Input: part model. Units: mm. Frame: model coordinates. A direction names the side the tool comes from. Give positions to 0.01 mm unless a question says otherwise; leave off trailing zeros. Write each loop counter-clockwise with the first axis right and the second up, starting at its lowest first coordinate (ties: lowest second). Pieces come first, ordered by that corner, then holes.
```python
from build123d import *

# Parameters (mm, degrees)
SKETCH_1_W          = 200
SKETCH_1_H          = 3
EXTRUDE_1_DEPTH     = 103
EXTRUDE_1_2_DEPTH   = 103
CHAMFER_1_SIZE      = 20
CHAMFER_2_SIZE      = 20
EXTRUDE_2_DEPTH     = 3
EXTRUDE_START       = 3
EXTRUDE_3_DEPTH     = 3
EXTRUDE_5_DEPTH     = 53
CUT_EXTRUDE_1_DEPTH = 45
EXTRUDE_START_2     = 53
EXTRUDE_6_DEPTH     = 53
CUT_EXTRUDE_START   = -45
CUT_EXTRUDE_3_DEPTH = 45
EXTRUDE_START_3     = 20
SKETCH_10_R         = 27
SKETCH_10_R_2       = 17
SKETCH_10_R_3       = 16.5
EXTRUDE_8_DEPTH     = 20
SKETCH_11_R         = 27
SKETCH_11_R_2       = 17
SKETCH_11_R_3       = 16.5
EXTRUDE_9_DEPTH     = 20
SKETCH_12_R         = 19
EXTRUDE_10_DEPTH    = 40
EXTRUDE_START_4     = 40
SKETCH_13_R         = 19
EXTRUDE_11_DEPTH    = 40


with BuildPart() as part:
    # Sketch 1 → Extrude 1 (new, symmetric)
    with BuildSketch(Plane(origin=(0, 0, 0), x_dir=(0, 0, -1), z_dir=(1, 0, 0))):
        Rectangle(SKETCH_1_W, SKETCH_1_H)
    extrude(amount=EXTRUDE_1_DEPTH, both=True)

    # Chamfer 2
    chamfer_2_edges = [part.edges().sort_by_distance(p)[0] for p in [
        (103, 0, 100),
        (103, 0, -100),
        (-103, 0, 100),
        (-103, 0, -100),
    ]]
    chamfer(chamfer_2_edges, length=CHAMFER_2_SIZE)



with BuildPart() as body_2:
    # Sketch 1 → Extrude 1 2 (new, symmetric)
    with BuildSketch(Plane(origin=(0, 0, 0), x_dir=(0, 0, -1), z_dir=(1, 0, 0))):
        with Locations((0, 45)):
            Rectangle(SKETCH_1_W, SKETCH_1_H)
    extrude(amount=EXTRUDE_1_2_DEPTH, both=True)

    # Chamfer 1
    chamfer_1_edges = [body_2.edges().sort_by_distance(p)[0] for p in [
        (103, 45, -100),
        (103, 45, 100),
        (-103, 45, -100),
        (-103, 45, 100),
    ]]
    chamfer(chamfer_1_edges, length=CHAMFER_1_SIZE)


with BuildPart() as part_1:
    add(part.part)

    add(body_2.part)  # Extrude 2 merges body 2
    # Sketch 2 → Extrude 2 (add)
    with BuildSketch(Plane(origin=(103, 0, 0), x_dir=(0, 0, -1), z_dir=(1, 0, 0))):
        with BuildLine():
            Line((105.840291615, 0.710043471), (31.760437422, 96.815065207))
            ThreePointArc((31.760437422, 96.815065207), (15.940085812, 107.430175203), (-3.082450225, 106.377935666))
            Line((-3.082450225, 106.377935666), (-177.38830015, 37.085290444))
            ThreePointArc((-177.38830015, 37.085290444), (-189.727961496, 21.787481591), (-183.015827469, 3.314867953))
            Line((-183.015827469, 3.314867953), (-148.015827469, -26.685132047))
            ThreePointArc((-148.015827469, -26.685132047), (-141.938924955, -30.257700298), (-135, -31.5))
            Line((-135, -31.5), (90, -31.5))
            ThreePointArc((90, -31.5), (107.947156731, -20.326073039), (105.840291615, 0.710043471))
        make_face()
    extrude(amount=EXTRUDE_2_DEPTH)

    # Sketch 3 → Extrude 3 (add)
    with BuildSketch(Plane.ZY.offset(103).offset(EXTRUDE_START)):
        with BuildLine():
            Line((-105.840291615, 0.710043471), (-31.760437422, 96.815065207))
            ThreePointArc((-31.760437422, 96.815065207), (-15.940085812, 107.430175203), (3.082450225, 106.377935666))
            Line((3.082450225, 106.377935666), (177.38830015, 37.085290444))
            ThreePointArc((177.38830015, 37.085290444), (189.727961496, 21.787481591), (183.015827469, 3.314867953))
            Line((183.015827469, 3.314867953), (148.015827469, -26.685132047))
            ThreePointArc((148.015827469, -26.685132047), (141.938924955, -30.257700298), (135, -31.5))
            Line((135, -31.5), (-90, -31.5))
            ThreePointArc((-90, -31.5), (-107.947156731, -20.326073039), (-105.840291615, 0.710043471))
        make_face()
    extrude(amount=-EXTRUDE_3_DEPTH)

    # Sketch 4 → Extrude 5 (add)
    with BuildSketch(Plane(origin=(106, 0, 0), x_dir=(0, 0, -1), z_dir=(1, 0, 0))):
        with BuildLine():
            Line((-3.082450225, 106.377935666), (-177.38830015, 37.085290444))
            ThreePointArc((-177.38830015, 37.085290444), (-189.727961496, 21.787481591), (-183.015827469, 3.314867953))
            Line((-183.015827469, 3.314867953), (-148.015827469, -26.685132047))
            ThreePointArc((-148.015827469, -26.685132047), (-141.938924955, -30.257700298), (-135, -31.5))
            Line((-135, -31.5), (90, -31.5))
            ThreePointArc((90, -31.5), (107.947156731, -20.326073039), (105.840291615, 0.710043471))
            Line((105.840291615, 0.710043471), (31.760437422, 96.815065207))
            ThreePointArc((31.760437422, 96.815065207), (15.940085812, 107.430175203), (-3.082450225, 106.377935666))
        make_face()
    extrude(amount=EXTRUDE_5_DEPTH)

    # Sketch 6 → Cut-Extrude 1 (cut)
    with BuildSketch(Plane(origin=(159, 0, 0), x_dir=(0, 0, -1), z_dir=(1, 0, 0))):
        with BuildLine():
            Line((-176.280055127, 34.297496878), (-1.974205202, 103.5901421))
            ThreePointArc((-1.974205202, 103.5901421), (15.146077231, 104.537157683), (29.38439368, 94.983558686))
            Line((29.38439368, 94.983558686), (103.464247872, -1.12146305))
            ThreePointArc((103.464247872, -1.12146305), (105.255083221, -19.002162083), (90, -28.5))
            Line((90, -28.5), (-135, -28.5))
            ThreePointArc((-135, -28.5), (-140.898086211, -27.444045253), (-146.063453349, -24.40736224))
            Line((-146.063453349, -24.40736224), (-181.063453349, 5.59263776))
            ThreePointArc((-181.063453349, 5.59263776), (-186.768767272, 21.294359353), (-176.280055127, 34.297496878))
        make_face()
    extrude(amount=-CUT_EXTRUDE_1_DEPTH, mode=Mode.SUBTRACT)

    # Sketch 8 → Extrude 6 (add)
    with BuildSketch(Plane.ZY.offset(106).offset(EXTRUDE_START_2)):
        with BuildLine():
            Line((-31.760437422, 96.815065207), (-105.840291615, 0.710043471))
            ThreePointArc((-105.840291615, 0.710043471), (-107.947156731, -20.326073039), (-90, -31.5))
            Line((-90, -31.5), (135, -31.5))
            ThreePointArc((135, -31.5), (141.938924955, -30.257700298), (148.015827469, -26.685132047))
            Line((148.015827469, -26.685132047), (183.015827469, 3.314867953))
            ThreePointArc((183.015827469, 3.314867953), (189.727961496, 21.787481591), (177.38830015, 37.085290444))
            Line((177.38830015, 37.085290444), (3.082450225, 106.377935666))
            ThreePointArc((3.082450225, 106.377935666), (-15.940085812, 107.430175203), (-31.760437422, 96.815065207))
        make_face()
    extrude(amount=-EXTRUDE_6_DEPTH)

    # Sketch 9 → Cut-Extrude 3 (cut)
    with BuildSketch(Plane.ZY.offset(159).offset(CUT_EXTRUDE_START)):
        with BuildLine():
            Line((-29.38439368, 94.983558686), (-103.464247872, -1.12146305))
            ThreePointArc((-103.464247872, -1.12146305), (-105.255083221, -19.002162083), (-90, -28.5))
            Line((-90, -28.5), (135, -28.5))
            ThreePointArc((135, -28.5), (140.898086211, -27.444045253), (146.063453349, -24.40736224))
            Line((146.063453349, -24.40736224), (181.063453349, 5.59263776))
            ThreePointArc((181.063453349, 5.59263776), (186.768767272, 21.294359353), (176.280055127, 34.297496878))
            Line((176.280055127, 34.297496878), (1.974205202, 103.5901421))
            ThreePointArc((1.974205202, 103.5901421), (-15.146077231, 104.537157683), (-29.38439368, 94.983558686))
        make_face()
    extrude(amount=CUT_EXTRUDE_3_DEPTH, mode=Mode.SUBTRACT)

    # Sketch 10 → Extrude 8 (add)
    with BuildSketch(Plane(origin=(114, 0, 0), x_dir=(0, 0, -1), z_dir=(1, 0, 0)).offset(EXTRUDE_START_3)):
        with Locations((8, 78.5)):
            Circle(SKETCH_10_R)
        with Locations((-170, 18.5)):
            Circle(SKETCH_10_R_2)
        with Locations((-135, -11.5)):
            Circle(SKETCH_10_R_2)
        with Locations((-60, -11.5)):
            Circle(SKETCH_10_R_3)
        with Locations((15, -11.5)):
            Circle(SKETCH_10_R_3)
        with Locations((90, -11.5)):
            Circle(SKETCH_10_R_2)
    extrude(amount=-EXTRUDE_8_DEPTH)

    # Sketch 11 → Extrude 9 (add)
    with BuildSketch(Plane.ZY.offset(114)):
        with Locations((-8, 78.5)):
            Circle(SKETCH_11_R)
        with Locations((-90, -11.5)):
            Circle(SKETCH_11_R_2)
        with Locations(Location((-15, -11.5, 0), (0, 0, 180))):
            Circle(SKETCH_11_R_3)
        with Locations(Location((60, -11.5, 0), (0, 0, 180))):
            Circle(SKETCH_11_R_3)
        with Locations((135, -11.5)):
            Circle(SKETCH_11_R_2)
        with Locations((170, 18.5)):
            Circle(SKETCH_11_R_2)
    extrude(amount=EXTRUDE_9_DEPTH)

    # Sketch 12 → Extrude 10 (add)
    with BuildSketch(Plane.ZY.offset(-103)):
        with Locations(Location((-8, 66.5, 0), (0, 0, 180))):
            Circle(SKETCH_12_R)
    extrude(amount=EXTRUDE_10_DEPTH)

    # Sketch 13 → Extrude 11 (add)
    with BuildSketch(Plane(origin=(-103, 0, 0), x_dir=(0, 0, -1), z_dir=(1, 0, 0)).offset(EXTRUDE_START_4)):
        with Locations((8, 66.5)):
            Circle(SKETCH_13_R)
    extrude(amount=-EXTRUDE_11_DEPTH)


solid = part_1.part
```
Q1. Mould query, pull axis X, two halves, no side actions, for faces 1 (the cylindrical face through (130.61, 22.07, 189.68)), 2 (the cylindrical face through (-82.72, 79.341, 6.004)), 3 (the flat face through (-134, -12, -15)), 4 (the flat face through (-103, 24, 42)). Classes: +X half, -X half, draft (parallel to the pull), parting line (faces both ways), or undercut.
Q2. Section B-B, the plane z = 88. Return the cut outline in (x, y), then the cut area to 3 significant figures.
Q3. Section A-A, the plane x = 36.5. Return the cut outline in (y, z), then the cut area to 3 significant figures.
Q4. Material intervals for line 1 along Y through (x, z) = (36, -33); line 2 along X through (y, z) = (50, 25); line 3 along X through (y, z) = (75, -46), sorted ascending.
Q5. Pin query (flat end, axial travel): pin 1 (2 mm diameter, centred on x = -102.5, z = 37.5, fed in from +Y); pin 2 (3 mm diameter, centred on y = 23, z = -38.5, fed in from +X); pin 3 (4 mm diameter, centred on x = 32, z = 38, fed in from +Y). Return the tip coordinate at first contact, or that it passes through.
Q6. Section D-D, the plane z = 170. Return the cut outline in (x, y), then the cut area to 3 significant figures.
Q7. Access query for faces 5 (the cylindrical face through (146.68, 104.6, -14.91)), 6 (the cylindrical face through (-146.32, 104.6, -14.91)), 7 (the flat face through (93, 0, 90)), 8 (the flat face through (1, 43.5, 1)). Directions: +Z, -Z, +X, -X, +Y, -Y. A direction counts if a zero-diameter tool reaches every point of the face in a straight line with its end or side. Return the directions, or none.
Solutions:
1. face 1: draft
1. face 2: undercut
1. face 3: -X half
1. face 4: undercut
2. outline: (-159, -31.5) - (-103, -31.5) - (-103, 72.62) - (-159, 72.62) - (-159, 69.39) - (-114, 69.39) - (-114, -28.5) - (-159, -28.5) - close; (-95, -1.5) - (95, -1.5) - (95, 1.5) - (-95, 1.5) - close; (-95, 43.5) - (95, 43.5) - (95, 46.5) - (-95, 46.5) - close; (103, -31.5) - (159, -31.5) - (159, -28.5) - (114, -28.5) - (114, 69.39) - (159, 69.39) - (159, 72.62) - (103, 72.62) - close
2. area: 3,990 mm2
3. outline: (-1.5, -100) - (1.5, -100) - (1.5, 100) - (-1.5, 100) - close; (43.5, -100) - (46.5, -100) - (46.5, 100) - (43.5, 100) - close
3. area: 1,200 mm2
4. line 1: y = -1.5 to 1.5, 43.5 to 46.5
4. line 2: x = -114 to -103, 103 to 114
4. line 3: x = -159 to -103, 103 to 159
5. pin 1: stops at y = 93.04
5. pin 2: stops at x = 114
5. pin 3: stops at y = 46.5
6. outline: (-159, -7.84) - (-103, -7.84) - (-103, 40.02) - (-159, 40.02) - (-159, 36.79) - (-114, 36.79) - (-114, 35.5) - (-134, 35.5) - (-134, 1.5) - (-114, 1.5) - (-114, -3.89) - (-159, -3.89) - close; (103, -7.84) - (159, -7.84) - (159, -3.89) - (114, -3.89) - (114, 1.5) - (134, 1.5) - (134, 35.5) - (114, 35.5) - (114, 36.79) - (159, 36.79) - (159, 40.02) - (103, 40.02) - close
6. area: 3,060 mm2
7. face 5: +X
7. face 6: -X
7. face 7: +Z, +Y, -Y
7. face 8: +Z, -Z
